Autodesk Inventor part; units mm, degrees
ref_plane "YZ Plane" through (0, 0, 0) normal (1, 0, 0) x (0, 1, 0)
ref_plane "XZ Plane" through (0, 0, 0) normal (0, 1, 0) x (-1, 0, 0)
ref_plane "XY Plane" through (0, 0, 0) normal (0, 0, 1) x (1, 0, 0)
sketch "スケッチ1" plane through (0, 0, 0) normal (0, 0, 1) x (1, 0, 0)
  line L0 (-9.75, 10.2) -> (9.75, 10.2)
  line L1 (9.75, 10.2) -> (9.75, 0)
  line L2 (9.75, 0) -> (-9.75, 0)
  line L3 (-9.75, 0) -> (-9.75, 10.2)
  line L4 (-9.75, 10.2) -> (9.75, 0) construction
  line L5 (9.75, 10.2) -> (-9.75, 0) construction
  line L6 (-13.65, 0) -> (13.65, 0)
  point P0 (0, 0)
  point P1 (0, 5.1)
  point P2 (0, 0)
  dimension "d0" = 19.5
  dimension "d1" = 10.2
extrude "押し出し1" add sketch "スケッチ1" along normal blind 3.2
sketch "スケッチ2" plane through (0, 0, 3.2) normal (0, 0, 1) x (1, 0, 0)
  line L0 (9.75, 0) -> (9.75, 10.2)
  line L1 (9.75, 0) -> (0, 0)
  line L2 (0, 0) -> (0, 9.5)
  line L3 (0, 9.5) -> (9.75, 9.5)
  line L4 (9.75, 9.5) -> (9.75, 0)
  line L5 (-9.75, 0) -> (9.75, 0)
  line L6 (0, 9.5) -> (-1.25, 10.2)
  line L7 (9.75, 10.2) -> (-9.75, 10.2)
  point P0 (0, 0)
  point P1 (0, 0)
  dimension "d4" = 9.5
  dimension "d5" = 11
extrude "押し出し2" cut sketch "スケッチ2" against normal through all contours L3 L6 L7 L0
sketch "スケッチ3" plane through (0, 0, 3.2) normal (0, 0, 1) x (1, 0, 0)
  circle A0 centre (-4.75, 2.5) radius 1.25
  circle A1 centre (4.75, 2.5) radius 1.25
  line L0 (0, -2.04) -> (0, 12.24)
  line L1 (-9.75, 0) -> (9.75, 0)
  point P0 (0, 0)
  dimension "d8" = 2.5
  dimension "d9" = 9.5
  dimension "d10" = 2.5
extrude "押し出し3" cut sketch "スケッチ3" against normal through all
sketch "スケッチ5" plane through (0, 0, 0) normal (0, 0, -1) x (-1, 0, 0)
  line L0 (9.75, 0) -> (-9.75, 0)
  line L1 (-0.25, 0) -> (0.25, 0)
  line L2 (0.25, 0) -> (0.25, -3.9)
  line L3 (0.25, -3.9) -> (-0.25, -3.9)
  line L4 (-0.25, -3.9) -> (-0.25, 0)
  line L5 (7.05, 0) -> (7.55, 0)
  line L6 (7.55, 0) -> (7.55, -3.9)
  line L7 (7.55, -3.9) -> (7.05, -3.9)
  line L8 (7.05, -3.9) -> (7.05, 0)
  line L9 (-7.55, 0) -> (-7.05, 0)
  line L10 (-7.05, 0) -> (-7.05, -3.9)
  line L11 (-7.05, -3.9) -> (-7.55, -3.9)
  line L12 (-7.55, -3.9) -> (-7.55, 0)
  line L13 (9.75, 0) -> (-9.75, 0)
  circle A0 centre (-4.75, 2.5) radius 1.25
  line L14 (-10.4269, 15) -> (-10.3503, 15.2901)
  line L15 (-10.3503, 15.2901) -> (7.8266, 10.4901)
  line L16 (7.8266, 10.4901) -> (7.75, 10.2)
  line L17 (7.75, 10.2) -> (-10.4269, 15)
  line L18 (-11.05, 10.2) -> (7.75, 10.2) construction
  line L19 (1.25, 10.2) -> (9.75, 10.2)
  circle A1 centre (4.75, 2.5) radius 1.25
  line L20 (9.75, 10.2) -> (9.75, 0)
  arc A2 (-10.4269, 15) -> (-11.05, 10.2) centre (7.75, 10.2) ccw construction
  circle A3 centre (-10.4269, 15) radius 1.3
  circle A4 centre (-10.4269, 15) radius 1.6
  line L21 (-10.4269, 15) -> (-11.9739, 15.4085)
  line L22 (7.8266, 10.4901) -> (8.925, 10.2)
  point P0 (0, 0)
  point P1 (7.3, -3.9)
  point P2 (0, -3.9)
  point P3 (-7.3, -3.9)
  point P4 (0, 0)
  point P5 (-8.8308, 14.8888)
  point P6 (-11.6838, 15.3319)
  point P7 (-9.17, 14.6681)
  dimension "d26" = 3.2
  dimension "d13" = 0.5
  dimension "d14" = 7.3
  dimension "d15" = 7.3
  dimension "d17" = 6.4
  dimension "d21" = 0.3
  dimension "d22" = 15.8
  dimension "d23" = 2
  dimension "d25" = 2.6
  dimension "d27" = 15
extrude "押し出し4" add sketch "スケッチ5" against normal blind 1.6 contours L10 L11 L12 L0 | L2 L3 L4 L0 | L6 L7 L8 L0 | L19 L16 L22 | L17 A4 L15 L16 | L17 A3 L15 A4 | L15 A3 L21 A4
mirror "ミラー1" about plane through (0, 5.1, 0) normal (0, 0, -1)
properties part number "limit_switch" material "アルミニウム 6061"
Check sheet for the modelled part. Datum: model origin and axes. Units: mm. A direction names the side the tool comes from. Coordinates: 2 decimals unless noted, no trailing zeros. Write each loop counter-clockwise with the first axis right and the second up, starting at its lowest first coordinate (ties: lowest second). Pieces come first, ordered by that corner, then holes.
Item 1: Mould release check, pull along X, two halves, no side actions. Record for faces 1 (the face through (-0.616, 9.845, 0.045)), 2 (the face through (-5.671, 1.655, -0.045)), 3 (the face through (-9.75, 5, 0)), 4 (the face through (0, 5, 3.2)): released by +X, released by -X, zero draft, split by the parting line, or undercut.
Numbers:
face 1: released by +X
face 2: undercut
face 3: released by -X
face 4: zero draft
Item 2: Cross-section at C-C on x = 4.25. Record the boundary of the cut face in (y, z), then the cut area to 3 significant figures.
Numbers:
outline: (0, -3.2) - (1.35, -3.2) - (1.35, 3.2) - (0, 3.2) - close; (3.65, -3.2) - (9.5, -3.2) - (9.5, 3.2) - (3.65, 3.2) - close; (13.37, -1.6) - (13.68, -1.6) - (13.68, 1.6) - (13.37, 1.6) - close
area: 47.1 mm2
Item 3: Cross-section at B-B on z = -2.5. Record the boundary of the cut face in (x, y).
Numbers:
outline: (-9.75, 0) - (9.75, 0) - (9.75, 9.5) - (0, 9.5) - (-1.25, 10.2) - (-9.75, 10.2) - close; hole circle Ø2.5 at (-4.75, 2.5); hole circle Ø2.5 at (4.75, 2.5)
Item 4: Scan lines: probe 1 along Y at (x, z) = (4.75, -0.25); probe 2 along Y at (x, z) = (-4.75, 1.25); probe 3 along Y at (x, z) = (4.25, 3). Record each from-to range of solid material in increasing order.
Numbers:
probe 1: y = 0 to 1.25, 3.75 to 9.5, 13.5 to 13.81
probe 2: y = 0 to 1.25, 3.75 to 10.2, 10.99 to 11.3
probe 3: y = 0 to 1.35, 3.65 to 9.5
Item 5: Cross-section at D-D on x = -8.5. Record the boundary of the cut face in (y, z).
Numbers:
outline: (0, -3.2) - (10.2, -3.2) - (10.2, -1.6) - (10.31, -1.6) - (10.31, 1.6) - (10.2, 1.6) - (10.2, 3.2) - (0, 3.2) - close
Item 6: Access from +Z, -Z, +X, -X, +Y, -Y to the whole of each face (thin tool, end or side, straight path). Record for faces 5 (the face through (5, 9.5, 0)), 6 (the face through (7.05, -2, 0)), 7 (the face through (-7.55, -2, 0)).
Numbers:
face 5: +Z, -Z, +X
face 6: +Z, -Z, -Y
face 7: +Z, -Z, -X, -Y
Item 7: Depth check by flat-ended pin: pin 1 Ø3 at (x, y) = (2.5, 13) entering from +Z; pin 2 Ø1 at (y, z) = (-1, 0) entering from -X; pin 3 Ø3 at (x, z) = (1.5, -1.5) entering from +Y. Enter the tip coordinate at first touch or a pass-through.
Numbers:
pin 1: stops at z = 1.6
pin 2: stops at x = -7.55
pin 3: stops at y = 13.35
Item 8: Cross-section at A-A on y = 2.5. Record the boundary of the cut face in (x, z), then the cut area to 3 significant figures.
Numbers:
outline: (-9.75, -3.2) - (-6, -3.2) - (-6, 3.2) - (-9.75, 3.2) - close; (-3.5, -3.2) - (3.5, -3.2) - (3.5, 3.2) - (-3.5, 3.2) - close; (6, -3.2) - (9.75, -3.2) - (9.75, 3.2) - (6, 3.2) - close
area: 92.8 mm2
